Read the model definition and answer for the solid it produces. Units are mm, in the model's axes. A direction names the side the tool comes from. Give positions to 0.01 mm unless a question says otherwise; leave off trailing zeros. Order: outer loops, then holes, each group sorted by start corner. A loop starts at its lowest first (then second) coordinate and runs counter-clockwise, first axis right, second up. Notation, with made-up numbers: M 56,51 L 86,51 A21 cw 86,60 Z; hole C 12.5,37 d4. An arc over 180 degrees is marked long. One line per item, written item: value.
from build123d import *

# Parameters (mm, degrees)
SKETCH1_W           = 40
SKETCH1_H           = 40
BOSS_EXTRUDE1_DEPTH = 5
SKETCH2_R           = 1.5
CUT_EXTRUDE1_DEPTH  = 2
SKETCH5_W           = 40
SKETCH5_H           = 10
BOSS_EXTRUDE2_DEPTH = 100
SKETCH6_W           = 40.003445824
SKETCH6_H           = 100
BOSS_EXTRUDE3_DEPTH = 7
SKETCH7_W           = 34
SKETCH7_H           = 31
CUT_EXTRUDE2_DEPTH  = 100
SKETCH8_W           = 3.001722912
SKETCH8_H           = 2
SKETCH8_H_2         = 2.093229538
BOSS_EXTRUDE4_DEPTH = 20


with BuildPart() as part:
    # Sketch1 → Boss-Extrude1 (new body)
    with BuildSketch(Plane(origin=(0, 0, 0), x_dir=(1, 0, 0), z_dir=(0, 1, 0))):
        with Locations((20, 20)):
            Rectangle(SKETCH1_W, SKETCH1_H)
    extrude(amount=BOSS_EXTRUDE1_DEPTH)

    # Sketch2 → Cut-Extrude1 (cut)
    with BuildSketch(Plane(origin=(0, 5, 0), x_dir=(1, 0, 0), z_dir=(0, 1, 0))):
        with Locations((10, 11.251726065)):
            Circle(SKETCH2_R)
        with Locations((30, 11.251726065)):
            Circle(SKETCH2_R)
    extrude(amount=-CUT_EXTRUDE1_DEPTH, mode=Mode.SUBTRACT)

    # Sketch5 → Boss-Extrude2 (add)
    with BuildSketch(Plane(origin=(0, 5, 0), x_dir=(1, 0, 0), z_dir=(0, 1, 0))):
        with Locations((20, 35)):
            Rectangle(SKETCH5_W, SKETCH5_H)
    extrude(amount=BOSS_EXTRUDE2_DEPTH)

    # Sketch6 → Boss-Extrude3 (add)
    with BuildSketch(Plane(origin=(0, 105, 0), x_dir=(1, 0, 0), z_dir=(0, 1, 0))):
        with Locations((20.001722912, 80)):
            Rectangle(SKETCH6_W, SKETCH6_H)
    extrude(amount=BOSS_EXTRUDE3_DEPTH)

    # Sketch7 → Cut-Extrude2 (cut)
    with BuildSketch(Plane(origin=(0, 112, 0), x_dir=(1, 0, 0), z_dir=(0, 1, 0))):
        with Locations((20.001722912, 112.5)):
            Rectangle(SKETCH7_W, SKETCH7_H)
    extrude(amount=-CUT_EXTRUDE2_DEPTH, mode=Mode.SUBTRACT)

    # Sketch8 → Boss-Extrude4 (add)
    with BuildSketch(Plane(origin=(0, 112, 0), x_dir=(1, 0, 0), z_dir=(0, 1, 0))):
        with Locations((38.502584368, 129)):
            Rectangle(SKETCH8_W, SKETCH8_H)
        with Locations((1.500861456, 129)):
            Rectangle(SKETCH8_W, SKETCH8_H)
        with Locations((1.500861456, 95.953385231)):
            Rectangle(SKETCH8_W, SKETCH8_H_2)
        with Locations((38.502584368, 95.953385231)):
            Rectangle(SKETCH8_W, SKETCH8_H_2)
    extrude(amount=BOSS_EXTRUDE4_DEPTH)


solid = part.part
1) Consider probe 1 along Z at (x, y) = (30, 4.4); probe 2 along Y at (x, z) = (36.5, -23); probe 3 along Y at (x, z) = (25, -66). Determine where each line is inside the solid, lowest interval first.
Reported:
probe 1: z = -40 to -12.75, -9.75 to 0
probe 2: y = 0 to 5
probe 3: y = 105 to 112
2) Find section C-C, the plane y = 97.5. Write down the section's boundary in (x, z).
Reported:
outline: M 0,-40 L 40,-40 L 40,-30 L 0,-30 Z
3) Each of these flat-tipped pins is pushed along its axis until it touches: pin 1 Ø12 at (x, y) = (5.5, 80.5) entering from +Z; pin 2 Ø3.5 at (x, y) = (1, 120) entering from +Z; pin 3 Ø3.5 at (x, z) = (38.5, -112) entering from +Y. Where does it stop, or does it pass through?
Reported:
pin 1: stops at z = -30
pin 2: stops at z = -94.91
pin 3: stops at y = 112
4) Find section A-A, the plane x = 19.5. Write down the section's boundary in (y, z).
Reported:
outline: M 0,-40 L 105,-40 L 105,-97 L 112,-97 L 112,-30 L 5,-30 L 5,0 L 0,0 Z; M 105,-130 L 112,-130 L 112,-128 L 105,-128 Z
5) Which of the six approach directions +Z, -Z, +X, -X, +Y, -Y give full straight-line access (tool end or side, diameter ignored) to faces 1 (the face through (38, 122, -97)), 2 (the face through (20, 5, -15)), 3 (the face through (30, 3, -11)), 4 (the face through (20, 109, -128))?
Reported:
face 1: +X, -X, +Y
face 2: +Z, +X, -X, +Y
face 3: +Y
face 4: +Y, -Y
6) Determine the mould class of faces 5 (the face through (20, 58, -30)), 6 (the face through (20, 112, -64)), 7 (the face through (37.002, 109, -112)) for opening direction Z: +Z half, -Z half, draft (parallel to the pull), parting line (faces both ways), or undercut.
Reported:
face 5: +Z half
face 6: draft
face 7: undercut
7) Find section B-B, the plane z = -108. Write down the section's boundary in (x, y), plus the area to 3 significant figures.
Reported:
outline: M 0,105 L 3,105 L 3,112 L 0,112 Z; M 37,105 L 40,105 L 40,112 L 37,112 Z
area: 42.0 mm^2
8) Find section D-D, the plane z = -23.5. Write down the section's boundary in (x, y).
Reported:
outline: M 0,0 L 40,0 L 40,5 L 0,5 Z
